Read the model definition and answer for the solid it produces. Units are mm, in the model's axes. Face numbers are marked on the shaded views. Coordinates: 2 decimals unless noted, no trailing zeros. Loops run counter-clockwise (first coordinate to the right, second up) from the corner with the lowest first, then second, coordinate; pieces in that order, holes last.
Q1. Section B-B (y = -21) is taken. Give the vertices of the cut face in (x, z).
Q2. Section A-A (z = 0) is taken. Give the vertices of the cut face in (x, y), then the cut area to 3 significant figures.
Q3. Section D-D (x = 0) is taken. Give the vertices of the cut face in (y, z).
Q4. The mould has two halves that part along Z. Classify the marked faces 1, 2 and 3: pulls with the +Z half, pulls with the -Z half, needs draft (parallel to the pull), parting line crosses it, or undercut.
Q5. Flat-ended cylindrical pins translate along their axes: P1, Ø2, axis at y = -7, z = -12, coming from the +X side; P2, Ø1.5, axis at x = -15.5, y = -29, coming from the +Z side; P3, Ø2, axis at x = 7.5, y = -23, coming from the +Z side; P4, Ø18, axis at x = 0, z = -47.41, coming from the +Y side. Find the tip coordinate at first contact, or state that the pin passes through.
Q6. Straight lines are drawn through the part: line 1 (X direction, y = -20.5, z = 0); line 2 (Z direction, x = 0, y = -23); line 3 (X direction, y = -26.5, z = 13). For each, find the intervals that lie inside material, in ascending order.
Q7. Section C-C (x = -22) is taken. Give the vertices of the cut face in (y, z).
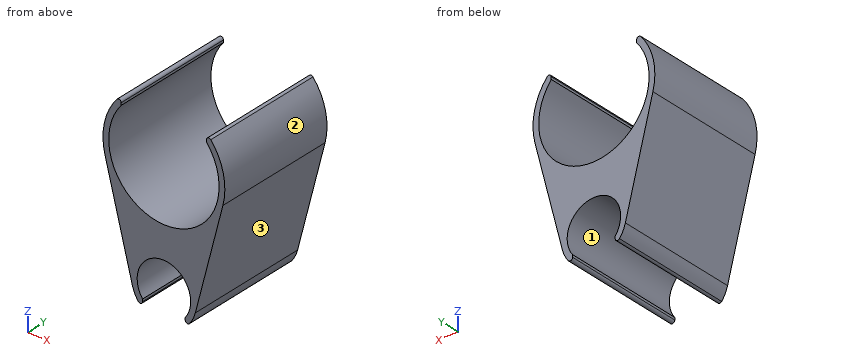
from build123d import *

# Parameters (mm, degrees)
F1_DEPTH = 50.8
F2_R     = 23
F2_R_2   = 11.1466666667
F3_DEPTH = 50.801
F5_DEPTH = 50.801
F6_R     = 1


with BuildPart() as f1:
    # F0 (on Front) → F1 (new body)
    with BuildSketch(Plane.XZ):
        with BuildLine():
            ThreePointArc((24.5934442484, -6.35), (0, 25.4), (-24.5934442484, -6.35))
            Line((-24.5934442484, -6.35), (-13.1165035992, -50.8))
            ThreePointArc((-13.1165035992, -50.8), (0, -60.96), (13.1165035992, -50.8))
            Line((13.1165035992, -50.8), (24.5934442484, -6.35))
        make_face()
    extrude(amount=F1_DEPTH)

    # F2 (on face) → F3 (cut, through all)
    with BuildSketch(Plane.XZ.offset(50.8)):
        Circle(F2_R)
        with Locations((0, -47.4133333333)):
            Circle(F2_R_2)
    extrude(amount=-F3_DEPTH, mode=Mode.SUBTRACT)

    # F4 (on face) → F5 (cut, through all)
    with BuildSketch(Plane.XZ.offset(50.8)):
        with BuildLine():
            ThreePointArc((-17.78, 14.5901199447), (0, 23), (17.78, 14.5901199447))
            Line((17.78, 14.5901199447), (17.78, 18.1392282085))
            ThreePointArc((17.78, 18.1392282085), (0, 25.4), (-17.78, 18.1392282085))
            Line((-17.78, 18.1392282085), (-17.78, 14.5901199447))
        make_face()
        with BuildLine():
            ThreePointArc((-8.89, -57.6348830093), (0, -60.96), (8.89, -57.6348830093))
            Line((8.89, -57.6348830093), (8.89, -54.1376234652))
            ThreePointArc((8.89, -54.1376234652), (0, -58.56), (-8.89, -54.1376234652))
            Line((-8.89, -54.1376234652), (-8.89, -57.6348830093))
        make_face()
    extrude(amount=-F5_DEPTH, mode=Mode.SUBTRACT)

    # F6
    f6_edges = [f1.edges().sort_by_distance(p)[0] for p in [
        (17.78, -25.4, 18.139228),
        (-17.78, -25.4, 18.139228),
        (8.89, -25.4, -57.634883),
        (-8.89, -25.4, -57.634883),
    ]]
    fillet(f6_edges, radius=F6_R)


solid = f1.part
Numbers:
1. outline: (-24.59, -6.35) - (-13.12, -50.8) arc R13.55 ccw to (-10.68, -55.75) arc R1 ccw to (-8.89, -55.13) - (-8.89, -54.14) arc R11.15 cw (long way) to (8.89, -54.14) - (8.89, -55.13) arc R1 ccw to (10.68, -55.75) arc R13.55 ccw to (13.12, -50.8) - (24.59, -6.35) arc R25.4 ccw to (19.55, 16.22) arc R1 ccw to (17.78, 15.58) - (17.78, 14.59) arc R23 cw (long way) to (-17.78, 14.59) - (-17.78, 15.58) arc R1 ccw to (-19.55, 16.22) arc R25.4 ccw to start
2. outline: (-25.4, -50.8) - (-23, -50.8) - (-23, 0) - (-25.4, 0) - close; (23, -50.8) - (25.4, -50.8) - (25.4, 0) - (23, 0) - close
2. area: 244 mm2
3. outline: (-50.8, -36.27) - (0, -36.27) - (0, -23) - (-50.8, -23) - close
4. face 1: undercut
4. face 2: parting line crosses it
4. face 3: pulls with the -Z half
5. P1: stops at x = 23.39
5. P2: stops at z = -16.28
5. P3: stops at z = -21.37
5. P4: passes through
6. line 1: x = -25.4 to -23, 23 to 25.4
6. line 2: z = -36.27 to -23
6. line 3: x = -21.82 to -18.97, 18.97 to 21.82
7. outline: (-50.8, -16.39) - (0, -16.39) - (0, -6.71) - (-50.8, -6.71) - close; (-50.8, 6.71) - (0, 6.71) - (0, 12.69) - (-50.8, 12.69) - close
